The listing builds one solid part. Answer for the finished solid, in the listing's coordinates (mm). Face numbers are marked on the shaded views. A direction names the side the tool comes from. Coordinates: 2 decimals unless noted, no trailing zeros. Order: outer loops, then holes, each group sorted by start corner. A loop starts at its lowest first (then second) coordinate and runs counter-clockwise, first axis right, second up. Notation, with made-up numbers: M 31,3.5 L 78,3.5 A21 ccw 78,39.5 Z; hole C 15.25,-12 d5. An arc over 180 degrees is marked long. One line per item, written item: value. Start each with the question number.
Q1. The part is cut by section C-C on z = 5.25. Give the vertices of the cut face in (x, y), then the cut area to 3 significant figures.
Q2. The part is cut by section B-B on y = -12.5. Give the vertices of the cut face in (x, z), then the cut area to 3 significant figures.
Q3. Each of these flat-tipped pins is pushed along its axis until it touches: pin 1 Ø1.2 at (y, z) = (6.5, -0.5) entering from +X; pin 2 Ø1.6 at (y, z) = (-8, -1) entering from +X; pin 3 Ø5 at (x, y) = (0.5, -1) entering from +Z; pin 4 Ø1.8 at (x, y) = (0, -12.5) entering from +Z. Where does it stop, or does it pass through?
Q4. The part is cut by section D-D on x = -5.5. Give the vertices of the cut face in (y, z).
Q5. Straight lines are drawn through the part: line 1 along Y through (x, z) = (0, 0.2); line 2 along X through (y, z) = (-2, 0.75); line 3 along Y through (x, z) = (0, 8.75). For each, find the intervals that lie inside material, in ascending order. Write a range as [from, to].
Q6. For the marked faces 4 and 5, determine the directions among +Z, -Z, +X, -X, +Y, -Y from which every point of the face is accessible in a straight line to the end or side of a thin tool.
Q7. The part is cut by section A-A on z = 2. Give the vertices of the cut face in (x, y).
Q8. Determine the mould class of the marked faces 1, 2 and 3 for opening direction X: pulls with the +X half, pulls with the -X half, needs draft (parallel to the pull), parting line crosses it, or undercut.
```python
from build123d import *

# Parameters (mm, degrees)
BOSS_EXTRU_1_DEPTH           = 8
BOSS_EXTRU_1_DEPTH_BACK      = 17
ENL_V_MAT_EXTRU_1_DEPTH      = 22.836729465
ENL_V_MAT_EXTRU_1_DEPTH_BACK = 22.836729465
ESQUISSE2_R                  = 2.5
ENL_V_START                  = 4
ESQUISSE3_R                  = 6
ENL_V_MAT_EXTRU_2_DEPTH      = 18.283796654
ESQUISSE5_W                  = 1.5
ESQUISSE5_H                  = 4
ENL_V_MAT_EXTRU_3_DEPTH      = 23.273807488
ESQUISSE6_R                  = 4.5
BOSS_EXTRU_2_DEPTH           = 1
BOSS_EXTRU_2_TAPER           = 45
ESQUISSE7_R                  = 1.5
ENL_V_MAT_EXTRU_4_DEPTH      = 23.566568193
CONG_1_R                     = 2
ENL_V_MAT_EXTRU_5_DEPTH      = 26.806975801


with BuildPart() as part:
    # Esquisse1 → Boss.-Extru.1 (new, two sides: drawn at the far end of the back side and taken through both)
    with BuildSketch(Plane(origin=(0, 0, 0), x_dir=(1, 0, 0), z_dir=(0, 1, 0)).offset(-BOSS_EXTRU_1_DEPTH_BACK)):
        Polygon((2.35, 0), (8, 0), (8, -10), (-8, -10), (-8, 0), (-2.35, 0), (-2.35, 1.5), (2.35, 1.5), align=None)
    extrude(amount=BOSS_EXTRU_1_DEPTH + BOSS_EXTRU_1_DEPTH_BACK)

    # Esquisse2 → Enlèv. mat.-Extru.1 (cut, two sides: drawn at the far end of the back side and taken through both)
    with BuildSketch(Plane(origin=(-1.372446517, 0, 0), x_dir=(1, 0, 0), z_dir=(0, 0, 1)).offset(-ENL_V_MAT_EXTRU_1_DEPTH_BACK)):
        with Locations((1.372446517, 0)):
            Circle(ESQUISSE2_R)
    extrude(amount=ENL_V_MAT_EXTRU_1_DEPTH + ENL_V_MAT_EXTRU_1_DEPTH_BACK, mode=Mode.SUBTRACT)

    # Esquisse3 → Enlèv. mat.-Extru.2 (cut, through all)
    with BuildSketch(Plane.XY.offset(ENL_V_START)):
        Circle(ESQUISSE3_R)
    extrude(amount=ENL_V_MAT_EXTRU_2_DEPTH, mode=Mode.SUBTRACT)

    # Esquisse5 → Enlèv. mat.-Extru.3 (cut, through all)
    with BuildSketch(Plane.ZY.offset(2.35)):
        with Locations((-0.75, 0)):
            Rectangle(ESQUISSE5_W, ESQUISSE5_H)
    extrude(amount=-ENL_V_MAT_EXTRU_3_DEPTH, mode=Mode.SUBTRACT)

    # Esquisse6 → Boss.-Extru.2 (add)
    with BuildSketch(Plane.XY.offset(10)):
        with Locations((0, -12.5)):
            Circle(ESQUISSE6_R)
    extrude(amount=BOSS_EXTRU_2_DEPTH, taper=BOSS_EXTRU_2_TAPER)

    # Esquisse7 → Enlèv. mat.-Extru.4 (cut, through all)
    with BuildSketch(Plane.XY.offset(11)):
        with Locations((0, -12.5)):
            Circle(ESQUISSE7_R)
    extrude(amount=-ENL_V_MAT_EXTRU_4_DEPTH, mode=Mode.SUBTRACT)

    # Congé1
    cong_1_edges = [part.edges().sort_by_distance(p)[0] for p in [
        (-8, -17, 5),
        (8, -17, 5),
        (-8, 8, 5),
        (8, 8, 5),
    ]]
    fillet(cong_1_edges, radius=CONG_1_R)

    # Esquisse8 → Enlèv. mat.-Extru.5 (cut, through all)
    with BuildSketch(Plane.ZY.offset(8)):
        Polygon((3, 8), (10, -8), (10, 8), align=None)
    extrude(amount=-ENL_V_MAT_EXTRU_5_DEPTH, mode=Mode.SUBTRACT)


solid = part.part
```
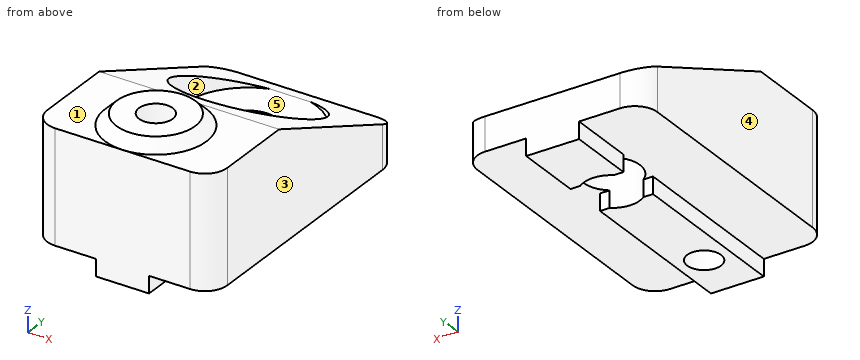
Output:
1. outline: M -8,-15 A2 ccw -6,-17 L 6,-17 A2 ccw 8,-15 L 8,2.86 L 5.28,2.86 A6 cw long -5.28,2.86 L -8,2.86 Z; hole C 0,-12.5 d3
1. area: 219 mm^2
2. outline: M -8,0 L -2.35,0 L -2.35,-1.5 L -1.5,-1.5 L -1.5,11 L -3.5,11 L -4.5,10 L -8,10 Z; M 1.5,-1.5 L 2.35,-1.5 L 2.35,0 L 8,0 L 8,10 L 4.5,10 L 3.5,11 L 1.5,11 Z
2. area: 138 mm^2
3. pin 1: stops at x = 7.99
3. pin 2: stops at x = 2.35
3. pin 3: stops at z = 4
3. pin 4: passes through
4. outline: M -17,0 L 8,0 L 8,3 L 2.4,5.45 L 2.4,4 L -2.4,4 L -2.4,7.55 L -8,10 L -17,10 Z
5. line 1: y = [-17, -14], [-11, -2.5], [2.5, 8]
5. line 2: x = [-8, -1.5], [1.5, 8]
5. line 3: y = [-17, -14], [-11, -6]
6. face 4: +Z, -Z, -X, +Y, -Y
6. face 5: +Z
7. outline: M -8,-15 A2 ccw -6,-17 L 6,-17 A2 ccw 8,-15 L 8,6 A2 ccw 6,8 L -6,8 A2 ccw -8,6 Z; hole C 0,0 d5; hole C 0,-12.5 d3
8. face 1: needs draft
8. face 2: undercut
8. face 3: pulls with the +X half
